```python
from build123d import *

# Parameters (mm, degrees)
SKETCH1_R           = 2.95
SKETCH1_R_2         = 1
BOSS_EXTRUDE1_DEPTH = 3
SKETCH2_R           = 4.5
SKETCH2_R_2         = 1
BOSS_EXTRUDE2_DEPTH = 5.5
SKETCH3_R           = 3.1
CUT_EXTRUDE1_DEPTH  = 3.25
CHAMFER1_SIZE       = 0.5
CHAMFER2_SIZE       = 0.5
SKETCH4_R           = 3.45
SKETCH4_R_2         = 1
BOSS_EXTRUDE3_DEPTH = 0.5
CHAMFER3_SIZE       = 1


with BuildPart() as part:
    # Sketch1 → Boss-Extrude1 (new body)
    with BuildSketch(Plane.XY):
        Circle(SKETCH1_R)
        Circle(SKETCH1_R_2, mode=Mode.SUBTRACT)
    extrude(amount=BOSS_EXTRUDE1_DEPTH)

    # Sketch2 → Boss-Extrude2 (add)
    with BuildSketch(Plane.XY.offset(3)):
        Circle(SKETCH2_R)
        Circle(SKETCH2_R_2, mode=Mode.SUBTRACT)
    extrude(amount=BOSS_EXTRUDE2_DEPTH)

    # Sketch3 → Cut-Extrude1 (cut)
    with BuildSketch(Plane.XY.offset(8.5)):
        Circle(SKETCH3_R)
    extrude(amount=-CUT_EXTRUDE1_DEPTH, mode=Mode.SUBTRACT)

    # Chamfer1
    chamfer1_edges = [part.edges().sort_by_distance(p)[0] for p in [
        (-3.1, 0, 8.5),
    ]]
    chamfer(chamfer1_edges, length=CHAMFER1_SIZE)

    # Chamfer2
    chamfer2_edges = [part.edges().sort_by_distance(p)[0] for p in [
        (-2.95, 0, 0),
    ]]
    chamfer(chamfer2_edges, length=CHAMFER2_SIZE)

    # Sketch4 → Boss-Extrude3 (add)
    with BuildSketch(Plane(origin=(0, 0, 3), x_dir=(-1, 0, 0), z_dir=(0, 0, -1))):
        Circle(SKETCH4_R)
        Circle(SKETCH4_R_2, mode=Mode.SUBTRACT)
    extrude(amount=BOSS_EXTRUDE3_DEPTH)

    # Chamfer3
    chamfer3_edges = [part.edges().sort_by_distance(p)[0] for p in [
        (-4.5, 0, 3),
    ]]
    chamfer(chamfer3_edges, length=CHAMFER3_SIZE)


solid = part.part
```
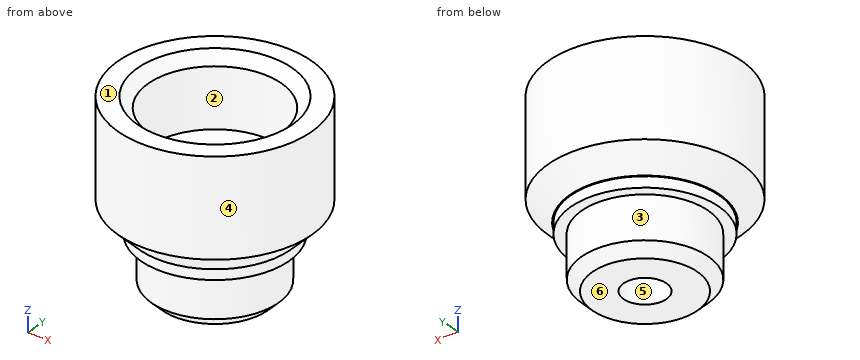
The listing builds one solid part. Answer for the finished solid, in the listing's coordinates (mm). Face numbers are marked on the shaded views. A direction names the side the tool comes from. Give positions to 0.01 mm unless a question says otherwise; leave off trailing zeros. Order: outer loops, then holes, each group sorted by start corner. A loop starts at its lowest first (then second) coordinate and runs counter-clockwise, first axis right, second up. Notation, with made-up numbers: (63.5, -37.5) -> (121.5, -37.5) arc R24 ccw to (121.5, -13.5) -> close; hole circle Ø4 at (9.25, -20.5). An arc over 180 degrees is marked (long way). Answer as a JSON object with one key per item and string values. Group by question number.
Item 1: Determine the mould class of the marked faces 4, 5 and 6 for opening direction Y: pulls with the +Y half, pulls with the -Y half, needs draft (parallel to the pull), parting line crosses it, or undercut.
Item 2: The part is cut by section A-A on x = 0. Write down the section's boundary in (y, z).
Item 3: Consider L1, parallel to Y at x = 0, z = 2.35; L2, parallel to X at y = -0.75, z = 8.25. Determine where each line is inside the solid, lowest interval first. Write a range as from..to.
Item 4: A tool of negligible diameter and unlimited length cuts with its end or side. For the marked faces 1, 2 and 3, from which of +Z, -Z, +X, -X, +Y, -Y can it reach the whole face along a straight path? Write none if from no direction.
Item 5: The part is cut by section C-C on z = 6. Write down the section's boundary in (x, y), and give its area (3 significant figures).
Item 6: Flat-ended cylindrical pins translate along their axes: pin 1 (2 mm diameter, centred on x = -3.5, y = -1, fed in from -Z); pin 2 (1 mm diameter, centred on y = 3, z = 2.5, fed in from +X); pin 3 (5 mm diameter, centred on x = 0, y = 0, fed in from -Z); pin 4 (1.5 mm diameter, centred on x = 0, y = 1, fed in from +Z). Find the tip coordinate at first contact, or state that the pin passes through.
Result set:
{
 "1": {"face 4": "parting line crosses it", "face 5": "undercut", "face 6": "needs draft"},
 "2": {"outline": "(-4.5, 4) -> (-3.5, 3) -> (-3.45, 3) -> (-3.45, 2.5) -> (-2.95, 2.5) -> (-2.95, 0.5) -> (-2.45, 0) -> (-1, 0) -> (-1, 5.25) -> (-3.1, 5.25) -> (-3.1, 8) -> (-3.6, 8.5) -> (-4.5, 8.5) -> close; (1, 0) -> (2.45, 0) -> (2.95, 0.5) -> (2.95, 2.5) -> (3.45, 2.5) -> (3.45, 3) -> (3.5, 3) -> (4.5, 4) -> (4.5, 8.5) -> (3.6, 8.5) -> (3.1, 8) -> (3.1, 5.25) -> (1, 5.25) -> close"},
 "3": {"L1": "-2.95..-1, 1..2.95", "L2": "-4.44..-3.26, 3.26..4.44"},
 "4": {"face 1": "+Z, +X, -X, +Y, -Y", "face 2": "+Z", "face 3": "-Z"},
 "5": {"outline": "circle Ø9 at (0, 0); hole circle Ø6.2 at (0, 0)", "area": "33.4 mm²"},
 "6": {"pin 1": "z = 0.19", "pin 2": "x = 2.38", "pin 3": "z = 0", "pin 4": "z = 5.25"}
}
